Verification items for the finished model (mm, model axes). Face numbers are marked on the shaded views. A direction names the side the tool comes from. Coordinates: 2 decimals unless noted, no trailing zeros. Write each loop counter-clockwise with the first axis right and the second up, starting at its lowest first coordinate (ties: lowest second). Pieces come first, ordered by that corner, then holes. Notation, with made-up numbers: (-19.5, 43) - (-13.5, 43) arc R11 ccw to (-13.5, 50) - close; hole circle Ø6 at (-5, 77.5). An arc over 180 degrees is marked (long way). Use one line per item in the form item = value. Start each with the question number.
(1) Sectioned sample at C-C (x = -5). Count the separate pieces of the cut face and the enclosed holes in it, and give its area (3 significant figures).
(2) Sectioned sample at A-A (y = -31). Record the cut outline in (x, z) (1 decimal).
(3) Material ranges on line 1 (X direction, y = -38.5, z = 17.5); line 2 (Y direction, x = -11, z = 14.5); line 3 (Z direction, x = -25, y = 6), recorded low to high. Write a range as [from, to].
(4) Gauge pin test, flat ends, axial feed: pin 1 Ø1.5 at (y, z) = (-45, 28.5) entering from -X; pin 2 Ø10 at (y, z) = (-22.5, 19.5) entering from -X; pin 3 Ø12 at (x, y) = (-48.5, -2.5) entering from +Z; pin 4 Ø4 at (x, z) = (-51.57, 17.14) entering from +Y. Record the tip position at first contact, or that the pin passes through.
(5) Tool access check on the marked faces 1, 2 and 3. Record the directions out of +Z, -Z, +X, -X, +Y, -Y that give a thin tool (end or side, any length) a straight path to the whole face; none if there is none.
(6) Sectioned sample at D-D (y = -9.5). Record the cut outline in (x, z).
(7) Sectioned sample at B-B (x = -32.5). Record the cut outline in (y, z) (3 decimals), and give its area (3 significant figures).
from build123d import *

# Parameters (mm, degrees)
F0_W      = 34.29
F0_H      = 34.29
F1_DEPTH  = 34.29
F2_R      = 12.7
F3_DEPTH  = 50.8
F4_R      = 12.7
F5_DEPTH  = 50.8
F6_R      = 3.429
F7_DEPTH  = 25.4
F8_R      = 3.429
F9_DEPTH  = 25.4
F10_R     = 3.429
F11_DEPTH = 25.4
F12_R     = 2.032
F13_R     = 2.54


with BuildPart() as f1:
    # F0 (on Top) → F1 (new body)
    with BuildSketch(Plane.XY):
        with Locations((3.6728888822, 6.5610635031)):
            Rectangle(F0_W, F0_H)
    extrude(amount=F1_DEPTH)

    # F2 (on face) → F3 (join)
    with BuildSketch(Plane(origin=(-13.4721111178, 0, 0), x_dir=(0, -1, 0), z_dir=(-1, 0, 0))):
        with Locations((-6.5610635031, 17.145)):
            Circle(F2_R)
    extrude(amount=F3_DEPTH)

    # F4 (on face) → F5 (join)
    with BuildSketch(Plane.XZ.offset(10.5839364969)):
        with Locations((3.6728888822, 17.145)):
            Circle(F4_R)
    extrude(amount=F5_DEPTH)

    # F6 (on Front) → F7 (cut, symmetric)
    with BuildSketch(Plane.XZ):
        with Locations((3.6728888822, 53.34)):
            Circle(F6_R)
        with Locations((3.6728888822, 72.39)):
            Circle(F6_R)
    extrude(amount=F7_DEPTH, both=True, mode=Mode.SUBTRACT)

    # F8 (on Right) → F9 (cut, symmetric)
    with BuildSketch(Plane.YZ):
        with Locations((-29.6339364969, 17.145)):
            Circle(F8_R)
        with Locations((-48.6839364969, 17.145)):
            Circle(F8_R)
    extrude(amount=F9_DEPTH, both=True, mode=Mode.SUBTRACT)

    # F10 (on Front) → F11 (cut, symmetric)
    with BuildSketch(Plane.XZ):
        with Locations((-51.5721111178, 17.145)):
            Circle(F10_R)
        with Locations((-32.5221111178, 17.145)):
            Circle(F10_R)
    extrude(amount=F11_DEPTH, both=True, mode=Mode.SUBTRACT)

    # F12
    f12_edges = [f1.edges().sort_by_distance(p)[0] for p in [
        (-9.027111, -61.383936, 17.145),
        (-64.272111, 19.261064, 17.145),
    ]]
    fillet(f12_edges, radius=F12_R)

    # F13
    f13_edges = [f1.edges().sort_by_distance(p)[0] for p in [
        (20.817889, 23.706064, 17.145),
        (20.817889, 6.561064, 34.29),
        (20.817889, -10.583936, 17.145),
        (20.817889, 6.561064, 0),
        (3.672889, 23.706064, 0),
        (3.672889, 23.706064, 34.29),
        (-13.472111, 23.706064, 17.145),
        (-13.472111, 6.561064, 0),
        (3.672889, -10.583936, 0),
        (-13.472111, 6.561064, 34.29),
        (-13.472111, -10.583936, 17.145),
        (3.672889, -10.583936, 34.29),
    ]]
    fillet(f13_edges, radius=F13_R)


solid = f1.part
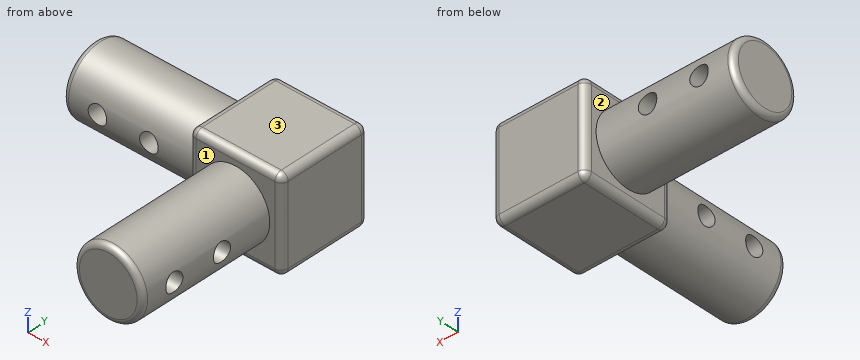
Answers below:
q1.separate_pieces = 1
q1.enclosed_holes = 2
q1.area = 2,040 mm2
q2.outline = (-8.6, 14) arc R12.7 ccw to (16, 14) - close; (-8.6, 20.3) - (16, 20.3) arc R12.7 ccw to start
q3.line_1 = [-9.02, 16.37]
q3.line_2 = [-10.58, 23.71]
q3.line_3 = [4.46, 29.83]
q4.pin_1 = -3.31
q4.pin_2 = -9.03
q4.pin_3 = 29.47
q4.pin_4 = through
q5.face_1 = -Y
q5.face_2 = -X
q5.face_3 = +Z, +X, -X, +Y, -Y
q6.outline = (-13.01, 2.54) arc R2.08 ccw to (-10.93, 0.46) - (18.28, 0.46) arc R2.08 ccw to (20.36, 2.54) - (20.36, 31.75) arc R2.08 ccw to (18.28, 33.83) - (-10.93, 33.83) arc R2.08 ccw to (-13.01, 31.75) - close
q7.outline = (-5.667, 13.716) arc R12.7 ccw to (18.789, 13.716) - close; (-5.667, 20.574) - (18.789, 20.574) arc R12.7 ccw to start
q7.area = 335 mm2
